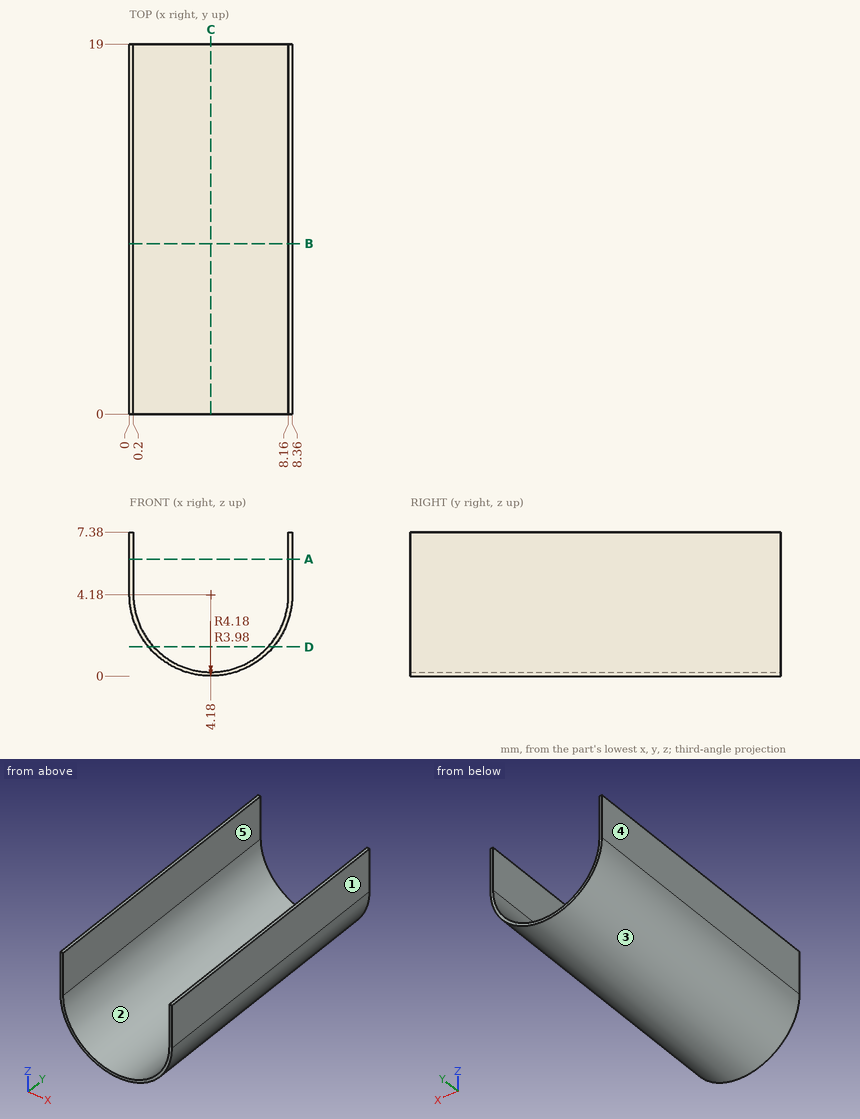
Input: dimensioned drawing with shaded views. Units: mm. Origin: part minimum x, y, z. A direction names the side the tool comes from. Coordinates: 2 decimals unless noted, no trailing zeros. Write each loop counter-clockwise with the first axis right and the second up, starting at its lowest first coordinate (ties: lowest second). Pieces come first, ordered by that corner, then holes. Notation, with made-up numbers: M 58,17 L 94,17 A23 cw 94,55 Z; hole C 13,29.5 d9. An arc over 180 degrees is marked long. Use a Markdown table: item, result.
1) Section A-A, the plane z = 6. Output: boundary loops of the cut face in (x, y).
Conclusion:
| item | result |
|---|---|
| outline | M 0,0 L 0.2,0 L 0.2,19 L 0,19 Z; M 8.16,0 L 8.36,0 L 8.36,19 L 8.16,19 Z |
2) Mould query, pull axis X, two halves, no side actions, for the marked faces 1, 2 and 3. Classes: pulls with the +X half, pulls with the -X half, needs draft (parallel to the pull), parting line crosses it, or undercut.
Conclusion:
| item | result |
|---|---|
| face 1 | pulls with the +X half |
| face 2 | undercut |
| face 3 | parting line crosses it |
3) Section C-C, the plane x = 4.18. Output: boundary loops of the cut face in (y, z), then the cut area to 3 significant figures.
Conclusion:
| item | result |
|---|---|
| outline | M 0,0 L 19,0 L 19,0.2 L 0,0.2 Z |
| area | 3.80 mm^2 |
4) Ray query, L1, parallel to X at y = 8.5, z = 6.5; L2, parallel to X at y = 15, z = 3.25; L3, parallel to Z at x = 3.75, y = 12. Return the intervals inside material, ascending.
Conclusion:
| item | result |
|---|---|
| L1 | x = 0 to 0.2, 8.16 to 8.36 |
| L2 | x = 0.1 to 0.31, 8.05 to 8.26 |
| L3 | z = 0.02 to 0.22 |
5) Section D-D, the plane z = 1.5. Output: boundary loops of the cut face in (x, y).
Conclusion:
| item | result |
|---|---|
| outline | M 0.97,0 L 1.24,0 L 1.24,19 L 0.97,19 Z; M 7.12,0 L 7.39,0 L 7.39,19 L 7.12,19 Z |
6) Reachability of the marked faces 4 and 5 from +Z, -Z, +X, -X, +Y, -Y: full face, straight path, thin tool, end or side. Return the list, or none.
Conclusion:
| item | result |
|---|---|
| face 4 | +Z, -Z, -X, +Y, -Y |
| face 5 | +Z, +Y, -Y |
7) First-contact query: pin 1 Ø1.5 at (x, y) = (1.5, 3) entering from +Z; pin 2 Ø3 at (x, y) = (5.5, 5) entering from +Z; pin 3 Ø2 at (x, y) = (6, 6) entering from -Z. Flat tips, straight axial feed; report the tip coordinate or a pass-through.
Conclusion:
| item | result |
|---|---|
| pin 1 | stops at z = 2.16 |
| pin 2 | stops at z = 1.37 |
| pin 3 | stops at z = 0.08 |
8) Section B-B, the plane y = 8.75. Output: boundary loops of the cut face in (x, z), then the cut area to 3 significant figures.
Conclusion:
| item | result |
|---|---|
| outline | M 0,4.18 A4.18 ccw 8.36,4.18 L 8.36,7.38 L 8.16,7.38 L 8.16,4.18 A3.98 cw 0.2,4.18 L 0.2,7.38 L 0,7.38 Z |
| area | 3.84 mm^2 |
